from build123d import *

# Parameters (mm, degrees)
SKETCH_1_W          = 76.4
SKETCH_1_H          = 2.1
SKETCH_1_W_2        = 79
SKETCH_1_H_2        = 1
EXTRUDE_1_DEPTH     = 100
SKETCH_2_R          = 0.35
CUT_EXTRUDE_1_DEPTH = 3
SKETCH_4_R          = 0.6
CUT_EXTRUDE_2_DEPTH = 108.563283698
SKETCH_4_3_R        = 1
CUT_EXTRUDE_3_DEPTH = 1.5
SKETCH_5_R          = 0.35
CUT_EXTRUDE_4_DEPTH = 108.563283698


with BuildPart() as part:
    # Sketch 1 → Extrude 1 (new body)
    with BuildSketch(Plane(origin=(0, 0, 0), x_dir=(0, 0, -1), z_dir=(1, 0, 0))):
        with Locations((0, -1.05)):
            Rectangle(SKETCH_1_W, SKETCH_1_H)
        with Locations((0, -2.6)):
            Rectangle(SKETCH_1_W_2, SKETCH_1_H_2)
    extrude(amount=EXTRUDE_1_DEPTH)

    # Sketch 2 → Cut-Extrude 1 (cut)
    with BuildSketch(Plane.ZY):
        with Locations((-13.8, -1.5)):
            Circle(SKETCH_2_R)
        with Locations((13.8, -1.5)):
            Circle(SKETCH_2_R)
    extrude(amount=-CUT_EXTRUDE_1_DEPTH, mode=Mode.SUBTRACT)

    # Sketch 4 → Cut-Extrude 2 (cut, through all)
    with BuildSketch(Plane(origin=(0, 0, 0), x_dir=(1, 0, 0), z_dir=(0, 1, 0))):
        with Locations(Location((98.5, -13.8, 0), (0, 0, 270))):
            Circle(SKETCH_4_R)
        with Locations(Location((98.5, 13.8, 0), (0, 0, 270))):
            Circle(SKETCH_4_R)
    extrude(amount=-CUT_EXTRUDE_2_DEPTH, mode=Mode.SUBTRACT)

    # Sketch 4_3 → Cut-Extrude 3 (cut)
    with BuildSketch(Plane(origin=(0, 0, 0), x_dir=(1, 0, 0), z_dir=(0, 1, 0))):
        with Locations(Location((98.5, -13.8, 0), (0, 0, 270))):
            Circle(SKETCH_4_3_R)
        with Locations(Location((98.5, 13.8, 0), (0, 0, 270))):
            Circle(SKETCH_4_3_R)
    extrude(amount=-CUT_EXTRUDE_3_DEPTH, mode=Mode.SUBTRACT)

    # Sketch 5 → Cut-Extrude 4 (cut, through all)
    with BuildSketch(Plane(origin=(0, 0, 0), x_dir=(1, 0, 0), z_dir=(0, 1, 0))):
        with Locations(Location((90, 3.95, 0), (0, 0, 270))):
            Circle(SKETCH_5_R)
        with Locations(Location((90, -3.95, 0), (0, 0, 270))):
            Circle(SKETCH_5_R)
    extrude(amount=-CUT_EXTRUDE_4_DEPTH, mode=Mode.SUBTRACT)


solid = part.part
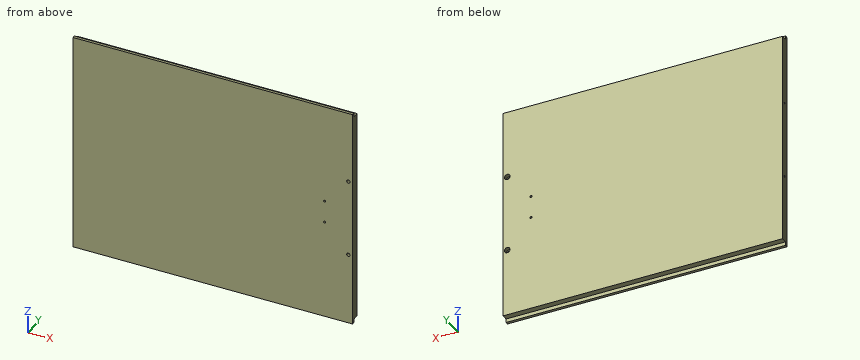
For this review, take the finished solid that the model builds, in its own axes (mm). Give positions to 0.01 mm unless a question says otherwise; leave off trailing zeros. Loops run counter-clockwise (first coordinate to the right, second up) from the corner with the lowest first, then second, coordinate; pieces in that order, holes last. Notation, with made-up numbers: M 53.25,51 L 89.25,51 A29 cw 89.25,82 Z; hole C -2,81 d4. An arc over 180 degrees is marked long. Put each result on its own line as item: value. Start each with the question number.
(1) Add section A-A, the plane x = 54. Write out the cut boundary in (y, z).
(2) For pin 1 (3 mm diameter, centred on x = 98.5, z = -13.8, fed in from +Y); pin 2 (1 mm diameter, centred on x = 98.5, z = -13.5, fed in from +Y); pin 3 (1.5 mm diameter, centred on x = 22, y = -0.5, fed in from +Z); pin 4 (1.4 mm diameter, centred on x = 64.5, z = 39, fed in from +Y), all flat-tipped, find the tip position at first contact; note any pin that passes through.
(3) Wall thickness on L1, parallel to Z at x = 90, y = -1.2; L2, parallel to Z at x = 98.5, y = -2.45; L3, parallel to X at y = -0.95, z = -13.8: over which ranges is each line inside the solid? List them lowest first.
Result:
1. outline: M -3.1,-39.5 L -2.1,-39.5 L -2.1,-38.2 L 0,-38.2 L 0,38.2 L -2.1,38.2 L -2.1,39.5 L -3.1,39.5 Z
2. pin 1: stops at y = 0
2. pin 2: stops at y = -1.5
2. pin 3: stops at z = 38.2
2. pin 4: stops at y = -2.1
3. L1: z = -38.2 to -4.3, -3.6 to 3.6, 4.3 to 38.2
3. L2: z = -39.5 to -14.4, -13.2 to 13.2, 14.4 to 39.5
3. L3: x = 0 to 97.5, 99.5 to 100
